Geometry: final body of the model. Coordinates: model frame, mm. Face numbers are marked on the shaded views. Give positions to 0.01 mm unless a question says otherwise; leave off trailing zeros. Write each loop counter-clockwise with the first axis right and the second up, starting at its lowest first coordinate (ties: lowest second). Pieces come first, ordered by that corner, then holes. Notation, with made-up numbers: M 8.5,2 L 66.5,2 A31 cw 66.5,27 Z; hole C 33,57.25 d7. An arc over 180 degrees is marked long. Answer as a JSON object with one key per item and string values.
Autodesk Inventor part; units mm, degrees
ref_plane "YZ Plane" through (0, 0, 0) normal (1, 0, 0) x (0, 1, 0)
ref_plane "XZ Plane" through (0, 0, 0) normal (0, 1, 0) x (-1, 0, 0)
ref_plane "XY Plane" through (0, 0, 0) normal (0, 0, 1) x (1, 0, 0)
sketch "Sketch1" plane through (0, 0, 0) normal (0, 0, 1) x (1, 0, 0)
  line L0 (-4.7625, -6.9215) -> (4.7625, -6.9215)
  line L1 (4.7625, -6.9215) -> (4.7625, 4.191)
  line L2 (4.7625, 4.191) -> (-4.7625, 4.191)
  line L3 (-4.7625, 4.191) -> (-4.7625, -6.9215)
  point P0 (0, 0)
  dimension "d0" = 9.525
  dimension "d1" = 11.1125
  dimension "d2" = 4.7625
  dimension "d3" = 4.191
extrude "Extrusion1" add sketch "Sketch1" along normal blind 12.7
sketch "Sketch2" plane through (0, 0, 12.7) normal (0, 0, 1) x (1, 0, 0)
  circle A0 centre (0, 0) radius 3.175
  dimension "d6" = 6.35
extrude "Extrusion2" cut sketch "Sketch2" against normal blind 7.62
sketch "Sketch3" plane through (0, 0, 5.08) normal (0, 0, 1) x (1, 0, 0)
  circle A0 centre (0, 0) radius 0.7937
  dimension "d9" = 1.5875
extrude "Extrusion3" add sketch "Sketch3" along normal blind 7.62
fillet "Fillet1" radius 0.7937 1 edges at (-0.7937, 0, 12.7)
properties part number "Plug"
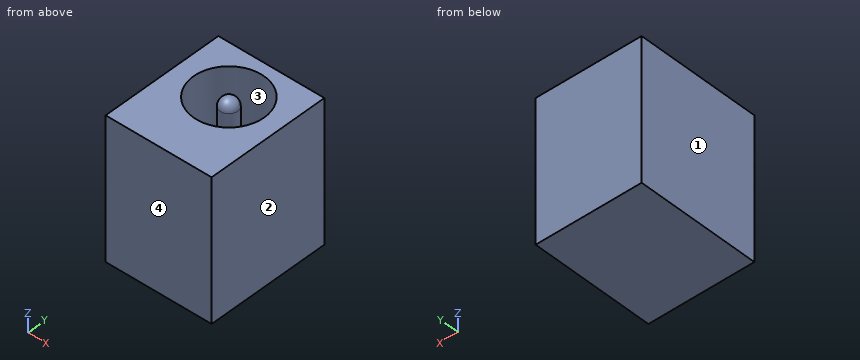
1) Pull-direction query (X, two-part tool) for the marked faces 1, 2, 3 and 4; classes: pulls with the +X half, pulls with the -X half, needs draft (parallel to the pull), parting line crosses it, or undercut.
Geometry check:
{"face 1": "pulls with the -X half", "face 2": "pulls with the +X half", "face 3": "undercut", "face 4": "needs draft"}
2) Cut plane C-C on y = 0. Return loops of the section in (x, z) (1 decimal), and give its area (3 significant figures).
Geometry check:
{"outline": "M -4.8,0 L 4.8,0 L 4.8,12.7 L 3.2,12.7 L 3.2,5.1 L 0.8,5.1 L 0.8,11.9 A0.8 ccw -0.8,11.9 L -0.8,5.1 L -3.2,5.1 L -3.2,12.7 L -4.8,12.7 Z", "area": "84.4 mm2"}
3) Cut plane A-A on z = 5.5. Give the number of separate pieces and of enclosed holes in the cut face, and give its area (3 significant figures).
Geometry check:
{"separate pieces": "2", "enclosed holes": "1", "area": "76.2 mm2"}
4) Line query: line 1 (Y direction, x = 0, z = 11) (1 decimal); line 2 (X direction, y = 1.25, z = 9.5); line 3 (Z direction, x = 0, y = 1). Output: solid intervals per line, ascending. Write a range as from..to.
Geometry check:
{"line 1": "y = -6.9..-3.2, -0.8..0.8, 3.2..4.2", "line 2": "x = -4.76..-2.92, 2.92..4.76", "line 3": "z = 0..5.08"}
5) Cut plane B-B on x = 0. Return loops of the section in (y, z) (1 decimal).
Geometry check:
{"outline": "M -6.9,0 L 4.2,0 L 4.2,12.7 L 3.2,12.7 L 3.2,5.1 L 0.8,5.1 L 0.8,11.9 A0.8 ccw -0.8,11.9 L -0.8,5.1 L -3.2,5.1 L -3.2,12.7 L -6.9,12.7 Z"}
6) Cut plane D-D on y = -2.75. Return loops of the section in (x, z), and give its area (3 significant figures).
Geometry check:
{"outline": "M -4.76,0 L 4.76,0 L 4.76,12.7 L 1.59,12.7 L 1.59,5.08 L -1.59,5.08 L -1.59,12.7 L -4.76,12.7 Z", "area": "96.8 mm2"}
